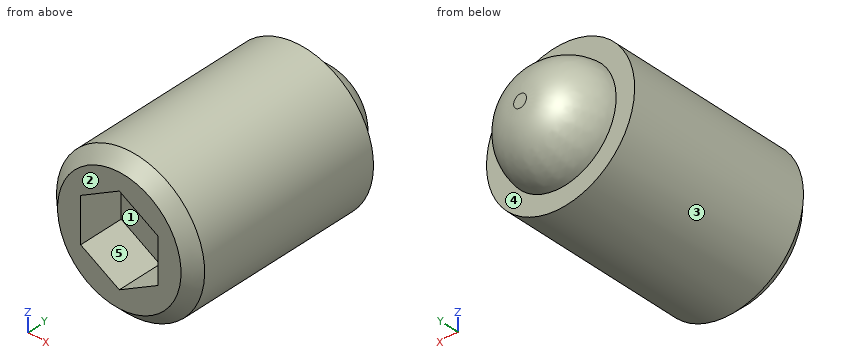
```python
from build123d import *

# Parameters (mm, degrees)
SKETCH_1_R          = 3
EXTRUDE_1_DEPTH     = 8
SKETCH_2_R          = 2.25
EXTRUDE_2_DEPTH     = 1.8
FILLET_2_R          = 2
CHAMFER_1_SIZE      = 0.5
CUT_EXTRUDE_1_DEPTH = 1.8


with BuildPart() as part:
    # 草图1 → 凸台-拉伸1 (new body)
    with BuildSketch(Plane(origin=(0, 0, 0), x_dir=(1, 0, 0), z_dir=(0, 1, 0))):
        with Locations(Location((0, 0, 0), (0, 0, 270))):
            Circle(SKETCH_1_R)
    extrude(amount=EXTRUDE_1_DEPTH)

    # 草图2 → 凸台-拉伸2 (add)
    with BuildSketch(Plane(origin=(0, 8, 0), x_dir=(1, 0, 0), z_dir=(0, 1, 0))):
        with Locations(Location((0, 0, 0), (0, 0, 270))):
            Circle(SKETCH_2_R)
    extrude(amount=EXTRUDE_2_DEPTH)

    # 圆角2
    # the kernel refuses this fillet: 2 mm, written as the material it takes off along each edge
    with BuildSketch(Plane(origin=(0, 9.8, 0), x_dir=(0, 0, 1), z_dir=(-1, 0, 0))) as fillet_2_piece_1:
        with BuildLine():
            CenterArc((0.260025126, -2), FILLET_2_R, 5.739170477, 84.260829523)
            Line((0.260025126, 0), (0.260025126, 0.04))
            Line((0.260025126, 0.04), (2.25, 0.04))
            Line((2.25, 0.04), (2.29, 0))
            ThreePointArc((2.29, 0), (2.29, -0.9), (2.289799497, -1.796))
            Line((2.289799497, -1.796), (2.25, -1.8))
        make_face()
    revolve(axis=Axis((0, 9.8, 0), (0, 1, 0)), mode=Mode.SUBTRACT)

    # 倒角1
    chamfer_1_edges = [part.edges().sort_by_distance(p)[0] for p in [
        (0, 0, -3),
    ]]
    chamfer(chamfer_1_edges, length=CHAMFER_1_SIZE)

    # 草图3 → 切除-拉伸1 (cut)
    with BuildSketch(Plane.XZ):
        Polygon((0, 1.808769012), (-1.566439914, 0.904384506), (-1.566439914, -0.904384506), (0, -1.808769012), (1.566439914, -0.904384506), (1.566439914, 0.904384506), align=None)
    extrude(amount=-CUT_EXTRUDE_1_DEPTH, mode=Mode.SUBTRACT)


solid = part.part
```
Build history of the part. All positions in model axes, mm. Face numbers are marked on the shaded views. A direction names the side the tool comes from. Coordinates: 2 decimals unless noted, no trailing zeros. Write each loop counter-clockwise with the first axis right and the second up, starting at its lowest first coordinate (ties: lowest second). Pieces come first, ordered by that corner, then holes.
1. Band-saw the part on A-A, the plane y = 4.5. Give the cut face in (x, z).
Answer block:
outline: circle Ø6 at (0, 0)
2. Drop flat-ended pins along their axis: pin 1 (1.6 mm diameter, centred on x = 0, z = 0, fed in from -Y); pin 2 (0.5 mm diameter, centred on y = 1, z = 0.5, fed in from +X); pin 3 (2 mm diameter, centred on y = 8, z = -2, fed in from +X). Give the stop position or say it passes through.
Answer block:
pin 1: stops at y = 1.8
pin 2: stops at x = 2.99
pin 3: stops at x = 2.83
3. 3-axis set-ups, long thin cutter, end or side, ignore diameter. For the marked faces 4 and 5: which of +Z, -Z, +X, -X, +Y, -Y reach the whole face in a straight line?
Answer block:
face 4: +Y
face 5: -Y
4. Pull direction Z, two halves, no side cores. Call the marked faces 1, 2 and 3: released by +Z, released by -Z, zero draft, split by the parting line, or undercut.
Answer block:
face 1: undercut
face 2: zero draft
face 3: split by the parting line
5. Drill centre lines: probe 1 along Z at (x, y) = (0.1, 4.25); probe 2 along Y at (x, z) = (-1.6, 2.25); probe 3 along Z at (x, y) = (-1, 1.5). Where is each one in solid material? Low to high.
Answer block:
probe 1: z = -3 to 3
probe 2: y = 0.26 to 8
probe 3: z = -2.83 to -1.23, 1.23 to 2.83
